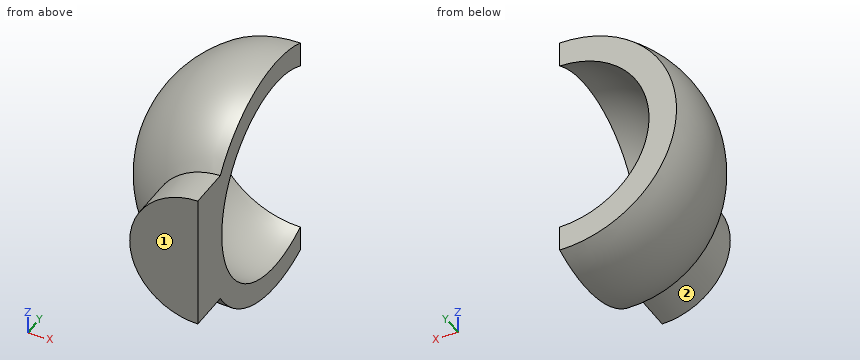
```python
from build123d import *

# Parameters (mm, degrees)
SKETCH2_W           = 42
SKETCH2_H           = 42
CUT_EXTRUDE1_DEPTH  = 20
SKETCH4_R           = 11
BOSS_EXTRUDE1_DEPTH = 3.5
SKETCH5_W           = 37.942079283
SKETCH5_H           = 42.029174216
CUT_EXTRUDE2_DEPTH  = 40


with BuildPart() as part:
    # Sketch1 → Revolve2 (revolve)
    with BuildSketch(Plane(origin=(0, 0, 0), x_dir=(1, 0, 0), z_dir=(0, 1, 0))):
        with BuildLine():
            Line((-20.31846942, 0), (19.68153058, 0))
            ThreePointArc((19.68153058, 0), (-0.31846942, 20), (-20.31846942, 0))
        make_face()
    revolve(axis=Axis((-66.656056584, 0, 0), (1, 0, 0)))

    # Sketch2 → Cut-Extrude1 (cut)
    with BuildSketch(Plane(origin=(0, 7.5, 0), x_dir=(1, 0, 0), z_dir=(0, 1, 0))):
        Rectangle(SKETCH2_W, SKETCH2_H)
    extrude(amount=CUT_EXTRUDE1_DEPTH, mode=Mode.SUBTRACT)

    # Sketch3 → Cut-Revolve1 (revolve, cut)
    with BuildSketch(Plane.XY):
        with BuildLine():
            Line((16.25, 0), (-16.25, 0))
            ThreePointArc((-16.25, 0), (0, -16.25), (16.25, 0))
        make_face()
    revolve(axis=Axis((-20.31846942, 0, 0), (1, 0, 0)), mode=Mode.SUBTRACT)

    # Sketch4 → Boss-Extrude1 (add, symmetric)
    with BuildSketch(Plane(origin=(0, -20, 0), x_dir=(1, 0, 0), z_dir=(0, 1, 0))):
        Circle(SKETCH4_R)
    extrude(amount=BOSS_EXTRUDE1_DEPTH, both=True)

    # Sketch5 → Cut-Extrude2 (cut)
    with BuildSketch(Plane.XZ.offset(23.5)):
        with Locations((18.971039642, 0)):
            Rectangle(SKETCH5_W, SKETCH5_H)
    extrude(amount=-CUT_EXTRUDE2_DEPTH, mode=Mode.SUBTRACT)


solid = part.part
```
Design review of the part built by this model. Coordinates are the model's own, in mm. Face numbers are marked on the shaded views. A direction names the side the tool comes from. Coordinates: 2 decimals unless noted, no trailing zeros. Order: outer loops, then holes, each group sorted by start corner. A loop starts at its lowest first (then second) coordinate and runs counter-clockwise, first axis right, second up. Notation, with made-up numbers: (88, 8) - (104, 8) arc R16 ccw to (104, 31) - close; hole circle Ø4 at (30.5, 87). An arc over 180 degrees is marked (long way). Answer in a Markdown table with one row per item.
(1) Consider section D-D on x = -4.5. State the section outline as (y, z) points.
Checked values:
| item | result |
|---|---|
| outline | (-23.5, -10.04) - (-16.79, -10.04) arc R19.56 ccw to (7.5, -18.06) - (7.5, -13.7) arc R15.61 cw (long way) to (7.5, 13.7) - (7.5, 18.06) arc R19.56 ccw to (-16.79, 10.04) - (-23.5, 10.04) - close |
(2) Consider section C-C on y = -21. State the section outline as (x, z) points.
Checked values:
| item | result |
|---|---|
| outline | (0, -11) - (0, 11) arc R11 ccw to start |
(3) Consider section B-B on z = -3.5. State the section outline as (x, y) points.
Checked values:
| item | result |
|---|---|
| outline | (-18.53, 7.5) arc R19.69 ccw to (-10.43, -16.9) - (-10.43, -23.5) - (0, -23.5) - (0, -15.87) arc R15.87 cw to (-13.98, 7.5) - close |
(4) For the marked faces 1 and 2, list the 3-axis set-ups (+Z, -Z, +X, -X, +Y, -Y) from which the entire face can be reached by the end or side of a thin tool; tool diameter is ignored.
Checked values:
| item | result |
|---|---|
| face 1 | +Z, -Z, +X, -X, -Y |
| face 2 | -X, -Y |
(5) Wall thickness on line 1 along Z through (x, y) = (-2.5, 1); line 2 along Y through (x, z) = (-14.25, 4.5); line 3 along Y through (x, z) = (-14.5, -2.5): over which ranges is each line inside the solid? List them lowest first. Write a range as from..to.
Checked values:
| item | result |
|---|---|
| line 1 | -19.86..-16.03, 16.03..19.86 |
| line 2 | -13.63..-6.38, 6.38..7.5 |
| line 3 | -13.88..-6.9, 6.9..7.5 |
(6) Consider section A-A on x = -8.5. State the section outline as (y, z) points.
Checked values:
| item | result |
|---|---|
| outline | (-23.5, -6.98) - (-16.86, -6.98) arc R18.25 ccw to (7.5, -16.64) - (7.5, -11.64) arc R13.85 cw (long way) to (7.5, 11.64) - (7.5, 16.64) arc R18.25 ccw to (-16.86, 6.98) - (-23.5, 6.98) - close |
(7) Clearance check with flat-ended pins moving along their axes: pin 1 (4 mm diameter, centred on x = -9.5, y = -8, fed in from -Z); pin 2 (4 mm diameter, centred on y = -8, z = 0, fed in from +X); pin 3 (10 mm diameter, centred on y = -19.5, z = -3.5, fed in from -X). State where each tip first meets the part, or that it passes through.
Checked values:
| item | result |
|---|---|
| pin 1 | z = -17.22 |
| pin 2 | x = -12.81 |
| pin 3 | x = -13.76 |
